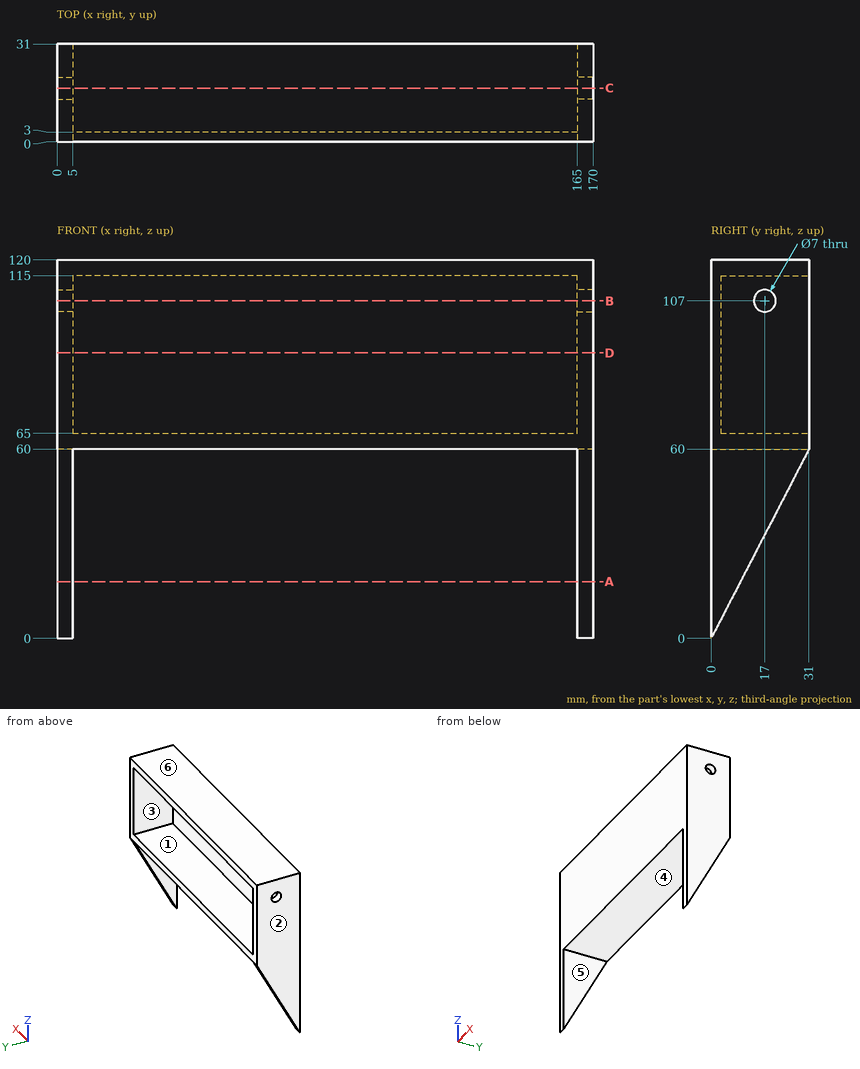
Input: dimensioned drawing with shaded views. Units: mm. Origin: part minimum x, y, z. A direction names the side the tool comes from. Coordinates: 2 decimals unless noted, no trailing zeros. Order: outer loops, then holes, each group sorted by start corner. A loop starts at its lowest first (then second) coordinate and runs counter-clockwise, first axis right, second up.
Item 1: Contact query for a flat-ended pin moving along its axis: P1, Ø8, axis at y = 17, z = 107, coming from the -X side. Output: stop coordinate, or through.
Answer:
P1: stops at x = 0
Item 2: Section query D-D (z = 90.5). Output: boundary loops of the cut face in (x, y).
Answer:
outline: (0, 0) - (170, 0) - (170, 31) - (165, 31) - (165, 3) - (5, 3) - (5, 31) - (0, 31) - close
Item 3: Access query for the marked faces 5 and 6. Directions: +Z, -Z, +X, -X, +Y, -Y. A direction counts if a zero-diameter tool reaches every point of the face in a straight line with its end or side. Return the directions, or none.
Answer:
face 5: -Z, +Y, -Y
face 6: +Z, +X, -X, +Y, -Y
Item 4: Section query B-B (z = 107). Output: boundary loops of the cut face in (x, y).
Answer:
outline: (0, 0) - (170, 0) - (170, 13.5) - (165, 13.5) - (165, 3) - (5, 3) - (5, 13.5) - (0, 13.5) - close; (0, 20.5) - (5, 20.5) - (5, 31) - (0, 31) - close; (165, 20.5) - (170, 20.5) - (170, 31) - (165, 31) - close
Item 5: Draft query along Z for the marked faces 1, 2, 3 and 4. Return one class per face: released by +Z, released by -Z, zero draft, split by the parting line, or undercut.
Answer:
face 1: undercut
face 2: zero draft
face 3: undercut
face 4: released by -Z
Item 6: Section query A-A (z = 18). Output: boundary loops of the cut face in (x, y), then the cut area to 3 significant figures.
Answer:
outline: (0, 0) - (5, 0) - (5, 9.3) - (0, 9.3) - close; (165, 0) - (170, 0) - (170, 9.3) - (165, 9.3) - close
area: 93.0 mm2
Item 7: Material intervals for line 1 along Y through (x, z) = (167.4, 107); line 2 along Z through (x, y) = (112.5, 25); line 3 along X through (y, z) = (12, 112), sorted ascending.
Answer:
line 1: y = 0 to 13.5, 20.5 to 31
line 2: z = 60 to 65, 115 to 120
line 3: x = 0 to 5, 165 to 170
Item 8: Section query C-C (y = 17). Output: boundary loops of the cut face in (x, z).
Answer:
outline: (0, 32.9) - (5, 32.9) - (5, 60) - (165, 60) - (165, 32.9) - (170, 32.9) - (170, 103.5) - (165, 103.5) - (165, 65) - (5, 65) - (5, 103.5) - (0, 103.5) - close; (0, 110.5) - (5, 110.5) - (5, 115) - (165, 115) - (165, 110.5) - (170, 110.5) - (170, 120) - (0, 120) - close
